Input: part model. Units: mm. Frame: model coordinates. A direction names the side the tool comes from. Round coordinates to 2 decimals unless told otherwise and drop trailing zeros. Order: outer loops, then holes, each group sorted by start corner. A loop starts at its lowest first (then second) coordinate and runs counter-clockwise, first axis right, second up. Notation, with made-up numbers: (78.5, 41.5) -> (107.5, 41.5) arc R24 cw to (107.5, 61.5) -> close; hole circle Ø3 at (-15.5, 77.25). An arc over 180 degrees is marked (long way). Answer as CSV lines item,"result". Start each with the question number.
1) Section query B-B, the plane x = 10. Output: boundary loops of the cut face in (y, z), and give its area (3 significant figures).
2) Line query: L1, parallel to Y at x = -15, z = -41; L2, parallel to Z at x = -18, y = 12; L3, parallel to Z at x = 14.5, y = -11. Output: solid intervals per line, ascending.
3) Mould query, pull axis Z, two halves, no side actions, for faces 1 (the face through (0.445, -12.093, 45.381)), 2 (the face through (1.38, -6.2, -78.79)), 3 (the face through (7, 0, 60.008)). Classes: +Z half, -Z half, draft (parallel to the pull), parting line (faces both ways), or undercut.
4) Section query A-A, the plane y = -12.7. Output: boundary loops of the cut face in (x, z).
5) Access query for faces 4 (the face through (0, 0, 21.908)), 5 (the face through (0, 0, -98.108)). Directions: +Z, -Z, +X, -X, +Y, -Y. A direction counts if a zero-diameter tool reaches every point of the face in a straight line with its end or side. Return the directions, or none.
6) Section query D-D, the plane y = 8. Output: boundary loops of the cut face in (x, z), and give its area (3 significant figures).
7) First-contact query: P1, Ø10, axis at x = 0, y = 0, coming from the +Z side; P2, Ø12, axis at x = -5.5, y = 21, coming from the -Z side. Flat tips, straight axial feed; report the tip coordinate or a pass-through.
8) Section query C-C, the plane z = 36. Output: boundary loops of the cut face in (x, y), and give its area (3 significant figures).
```python
from build123d import *

# Parameters (mm, degrees)
SKETCH1_W              = 63.5
SKETCH1_H              = 63.5
BOSS_EXTRUDE1_DEPTH    = 60.0075
SKETCH2_R              = 6.35
BOSS_EXTRUDE2_DEPTH    = 38.1
SKETCH3_R              = 6.35
CUT_EXTRUDE1_DEPTH     = 38.1
F_10_32_TAPPED_HOLE1_D = 4.0386


with BuildPart() as part:
    # Sketch1 → Boss-Extrude1 (new body, symmetric)
    with BuildSketch(Plane.XY):
        Rectangle(SKETCH1_W, SKETCH1_H)
    extrude(amount=BOSS_EXTRUDE1_DEPTH, both=True)

    # Sketch2 → Boss-Extrude2 (add)
    with BuildSketch(Plane(origin=(0, 0, -60.0075), x_dir=(-1, 0, 0), z_dir=(0, 0, -1))):
        Circle(SKETCH2_R)
    extrude(amount=BOSS_EXTRUDE2_DEPTH)

    # Sketch3 → Cut-Extrude1 (cut)
    with BuildSketch(Plane.XY.offset(60.0075)):
        Circle(SKETCH3_R)
    extrude(amount=-CUT_EXTRUDE1_DEPTH, mode=Mode.SUBTRACT)

    # #10-32 Tapped Hole1 (through all)
    with Locations(Plane.ZY.offset(31.75)):
        with Locations((-40.9575, 12.7), (-40.9575, -12.7), (47.3075, -12.7), (47.3075, 12.7)):
            Hole(F_10_32_TAPPED_HOLE1_D / 2)


solid = part.part
```
Findings:
1,outline,"(-31.75, -60.01) -> (31.75, -60.01) -> (31.75, 60.01) -> (-31.75, 60.01) -> close; hole circle Ø4.04 at (-12.7, -40.96); hole circle Ø4.04 at (-12.7, 47.31); hole circle Ø4.04 at (12.7, -40.96); hole circle Ø4.04 at (12.7, 47.31)"
1,area,"7,570 mm^2"
2,L1,"y = -31.75 to -14.72, -10.68 to 10.68, 14.72 to 31.75"
2,L2,"z = -60.01 to -42.85, -39.06 to 45.41, 49.2 to 60.01"
2,L3,"z = -60.01 to -42.05, -39.87 to 46.22, 48.4 to 60.01"
3,face 1,"undercut"
3,face 2,"draft"
3,face 3,"+Z half"
4,outline,"(-31.75, -60.01) -> (31.75, -60.01) -> (31.75, -42.98) -> (-31.75, -42.98) -> close; (-31.75, -38.94) -> (31.75, -38.94) -> (31.75, 45.29) -> (-31.75, 45.29) -> close; (-31.75, 49.33) -> (31.75, 49.33) -> (31.75, 60.01) -> (-31.75, 60.01) -> close"
5,face 4,"+Z"
5,face 5,"-Z, +X, -X, +Y, -Y"
6,outline,"(-31.75, -60.01) -> (31.75, -60.01) -> (31.75, 60.01) -> (-31.75, 60.01) -> close"
6,area,"7,620 mm^2"
7,P1,"stops at z = 21.91"
7,P2,"stops at z = -60.01"
8,outline,"(-31.75, -31.75) -> (31.75, -31.75) -> (31.75, 31.75) -> (-31.75, 31.75) -> close; hole circle Ø12.7 at (0, 0)"
8,area,"3,910 mm^2"
